```python
from build123d import *

# Parameters (mm, degrees)
F0_W      = 40
F0_H      = 20
F1_DEPTH  = 10
F2_R      = 1
F2_R_2    = 2.5
F2_R_3    = 1.5
F3_DEPTH  = 10
F4_R      = 1.5
F4_R_2    = 2
F4_R_3    = 2.5
F4_R_4    = 3
F4_R_5    = 1
F5_DEPTH  = 10
F6_W      = 10
F6_H      = 0.5
F7_DEPTH  = 20.001
F8_R      = 2.5
F9_DEPTH  = 9.501
F10_R     = 3.5
F10_R_2   = 2.5
F11_DEPTH = 3
F12_W     = 0.5
F12_H     = 2
F13_DEPTH = 10


with BuildPart() as f1:
    # F0 (on Top) → F1 (new body)
    with BuildSketch(Plane.XY):
        Rectangle(F0_W, F0_H)
    extrude(amount=F1_DEPTH)

    # F2 (on face) → F3 (cut)
    with BuildSketch(Plane(origin=(-20, 0, 0), x_dir=(0, -1, 0), z_dir=(-1, 0, 0))):
        with Locations((6, 5)):
            Circle(F2_R)
        with Locations((-5, 5)):
            Circle(F2_R_2)
        with Locations((1, 5)):
            Circle(F2_R_3)
    extrude(amount=-F3_DEPTH, mode=Mode.SUBTRACT)

    # F4 (on face) → F5 (cut)
    with BuildSketch(Plane.XZ.offset(10)):
        with Locations((-9, 5)):
            Circle(F4_R)
        with Locations((-3, 5)):
            Circle(F4_R_2)
        with Locations((4, 5)):
            Circle(F4_R_3)
        with Locations((12, 5)):
            Circle(F4_R_4)
        with Locations((-14, 5)):
            Circle(F4_R_5)
    extrude(amount=-F5_DEPTH, mode=Mode.SUBTRACT)

    # F6 (on face) → F7 (cut, through all)
    with BuildSketch(Plane.XZ.offset(10)):
        with Locations((15, 9.75)):
            Rectangle(F6_W, F6_H)
    extrude(amount=-F7_DEPTH, mode=Mode.SUBTRACT)

    # F8 (on face) → F9 (cut, through all)
    with BuildSketch(Plane.XY.offset(9.5)):
        with Locations((15, 4)):
            Circle(F8_R)
        with Locations((15, -4)):
            Circle(F8_R)
    extrude(amount=-F9_DEPTH, mode=Mode.SUBTRACT)

    # F10 (on face) → F11 (join)
    with BuildSketch(Plane.XY.offset(9.5)):
        with Locations((15, 4)):
            Circle(F10_R)
        with Locations((15, 4)):
            Circle(F10_R_2, mode=Mode.SUBTRACT)
    extrude(amount=F11_DEPTH)

    # F12 (on face) → F13 (join)
    with BuildSketch(Plane.YZ.offset(20)):
        with Locations((10.25, 8.5)):
            Rectangle(F12_W, F12_H)
    extrude(amount=-F13_DEPTH)


solid = f1.part
```
Check sheet for the modelled part. Datum: model origin and axes. Units: mm. A direction names the side the tool comes from. Coordinates: 2 decimals unless noted, no trailing zeros. Order: outer loops, then holes, each group sorted by start corner. A loop starts at its lowest first (then second) coordinate and runs counter-clockwise, first axis right, second up. Notation, with made-up numbers: M -18.5,-28.75 L 29.5,-28.75 A25 ccw 29.5,-3.75 Z; hole C 16,72.25 d4. An arc over 180 degrees is marked long. Write each question's results on one line, items separated by ' | '. Start each with the question number.
1. Cross-section at C-C on y = -8.5. Record the cut outline in (x, z), and give its area (3 significant figures).
2. Access from +Z, -Z, +X, -X, +Y, -Y to the whole of each face (thin tool, end or side, straight path). Record for faces 1 (the face through (18.233, 2.659, 10.979)), 2 (the face through (-10, 5, 5)), 3 (the face through (9, -5, 5)).
3. Cross-section at D-D on z = 11.5. Record the cut outline in (x, y), and give its area (3 significant figures).
4. Material ranges on probe 1 along Z at (x, y) = (-13, 5); probe 2 along Z at (x, y) = (-14, -7.5); probe 3 along X at (y, z) = (-4, 6.25), recorded low to high.
5. Mould release check, pull along Z, two halves, no side actions. Record for faces 4 (the face through (0, 0, 0)), 5 (the face through (0, 10, 5)), 6 (the face through (12, 0, 5)): +Z half, -Z half, draft (parallel to the pull), parting line (faces both ways), or undercut.
6. Go/stop test with flat-tipped pins: P1, Ø4, axis at x = 15, y = -4, coming from the -Z side; P2, Ø1.6, axis at x = -14, z = 5, coming from the -Y side; P3, Ø10, axis at x = 2.5, y = -2.5, coming from the +Z side; P4, Ø3, axis at x = -9.5, z = 6, coming from the +Y side. Record where each tip stops, or that it passes through.
7. Cross-section at A-A on y = -3. Record the cut outline in (x, z).
8. Cross-section at B-B on x = -3. Record the cut outline in (y, z).
Checks:
1) outline: M -20,0 L 20,0 L 20,9.5 L 10,9.5 L 10,10 L -20,10 Z; hole C -14,5 d2; hole C -9,5 d3; hole C -3,5 d4; hole C 4,5 d5; hole C 12,5 d6 | area: 324 mm²
2) face 1: +Z | face 2: -X | face 3: -Y
3) outline: C 15,4 d7; hole C 15,4 d5 | area: 18.8 mm²
4) probe 1: z = 0 to 2.5, 7.5 to 10 | probe 2: z = 0 to 4, 6 to 10 | probe 3: x = -20 to -9.83, -8.17 to -4.56, -1.44 to 1.83, 6.17 to 9.27, 17.5 to 20
5) face 4: -Z half | face 5: draft | face 6: undercut
6) P1: passes through | P2: stops at y = 0.27 | P3: stops at z = 10 | P4: stops at y = 10
7) outline: M -20,0 L 12.71,0 L 12.71,2.08 A3 cw long 12.71,7.92 L 12.71,9.5 L 10,9.5 L 10,10 L -20,10 Z; M 17.29,0 L 20,0 L 20,9.5 L 17.29,9.5 Z; hole C -14,5 d2; hole C -9,5 d3; hole C -3,5 d4; hole C 4,5 d5
8) outline: M -10,0 L 10,0 L 10,10 L -10,10 L -10,7 L 0,7 L 0,3 L -10,3 Z
